Check sheet for the modelled part. Datum: model origin and axes. Units: mm. A direction names the side the tool comes from. Round coordinates to 2 decimals unless told otherwise and drop trailing zeros. Order: outer loops, then holes, each group sorted by start corner. A loop starts at its lowest first (then second) coordinate and runs counter-clockwise, first axis right, second up.
Q1. Cross-section at A-A on z = -26. Record the cut outline in (x, y), then the cut area to 3 significant figures.
Q2. Mould release check, pull along X, two halves, no side actions. Record for faces 4 (the flat face through (21, 2, 32)), 5 (the flat face through (26, 1, 1)), 6 (the flat face through (-17, 1, 1)), 7 (the flat face through (-2, 3, -1)): +X half, -X half, draft (parallel to the pull), parting line (faces both ways), or undercut.
Q3. Cross-section at D-D on z = 3.5. Record the cut outline in (x, y).
Q4. Scan lines: probe 1 along X at (y, z) = (1.3, -31); probe 2 along X at (y, z) = (2.6, 32); probe 3 along X at (y, z) = (0.75, 15). Record each from-to range of solid material in increasing order.
Q5. Depth check by flat-ended pin: P1, Ø1.1, axis at x = -26, y = 2.5, coming from the -Z side; P2, Ø2.5, axis at x = 23, z = 33, coming from the -Y side; P3, Ø0.8, axis at y = 2.5, z = -31.5, coming from the -X side. Enter the tip coordinate at first touch or a pass-through.
Q6. Cross-section at C-C on y = 0.95. Record the cut outline in (x, z).
Q7. Set-up check for faces 1 (the cylindrical face through (3.138, 1.479, 11.853)), 2 (the flat face through (-23, 2, -1)), 3 (the cylindrical face through (24.27, 0.99, 30.23)): record each of +Z, -Z, +X, -X, +Y, -Y from which the full face is reachable in a straight line by a thin tool's end or side.
Q8. Cross-section at B-B on x = 15. Record the cut outline in (y, z).
from build123d import *

# Parameters (mm, degrees)
ESQUISSE1_R             = 1.7
ESQUISSE1_R_2           = 3.15
ESQUISSE1_R_3           = 1.4
BOSS_EXTRU_3_DEPTH      = 3
ESQUISSE1_5_R           = 1.4
ESQUISSE1_5_R_2         = 2.4
ENL_V_MAT_EXTRU_7_DEPTH = 2


with BuildPart() as part:
    # Esquisse1 → Boss.-Extru.3 (new body)
    with BuildSketch(Plane(origin=(0, 0, 0), x_dir=(1, 0, 0), z_dir=(0, 1, 0))):
        Polygon((-21, 36), (-21, 28), (-29, 28), (-29, -36), (26, -36), (26, 36), align=None)
        with Locations(Location((15, 31, 0), (0, 0, 270))):
            Circle(ESQUISSE1_R, mode=Mode.SUBTRACT)
        with Locations(Location((3, -15, 0), (0, 0, 270))):
            Circle(ESQUISSE1_R_2, mode=Mode.SUBTRACT)
        with Locations(Location((-15, 31, 0), (0, 0, 270))):
            Circle(ESQUISSE1_R, mode=Mode.SUBTRACT)
        with Locations(Location((-26.347888471, 26, 0), (0, 0, 270))):
            Circle(ESQUISSE1_R_3, mode=Mode.SUBTRACT)
        with Locations(Location((22.652111529, 26, 0), (0, 0, 270))):
            Circle(ESQUISSE1_R_3, mode=Mode.SUBTRACT)
        with Locations(Location((22.652111529, -32, 0), (0, 0, 270))):
            Circle(ESQUISSE1_R_3, mode=Mode.SUBTRACT)
        with Locations(Location((-26.347888471, -32, 0), (0, 0, 270))):
            Circle(ESQUISSE1_R_3, mode=Mode.SUBTRACT)
    extrude(amount=BOSS_EXTRU_3_DEPTH)

    # Esquisse1_5 → Enl_v. mat.-Extru.7 (cut)
    # profile 1 of 3: a face of its own
    with BuildSketch(Plane(origin=(0, 0, 0), x_dir=(1, 0, 0), z_dir=(0, 1, 0))):
        Polygon((-17, 36), (-21, 36), (-21, 28), (-29, 28), (-29, -36), (-17, -36), align=None)
        with Locations(Location((-26.347888471, 26, 0), (0, 0, 270))):
            Circle(ESQUISSE1_5_R, mode=Mode.SUBTRACT)
        with Locations(Location((-26.347888471, -32, 0), (0, 0, 270))):
            Circle(ESQUISSE1_5_R, mode=Mode.SUBTRACT)
    # profile 2 of 3: a face of its own
    with BuildSketch(Plane(origin=(0, 0, 0), x_dir=(1, 0, 0), z_dir=(0, 1, 0))):
        with Locations(Location((22.652111529, 26, 0), (0, 0, 270))):
            Circle(ESQUISSE1_5_R_2)
        with Locations(Location((22.652111529, 26, 0), (0, 0, 270))):
            Circle(ESQUISSE1_5_R, mode=Mode.SUBTRACT)
    # profile 3 of 3: a face of its own
    with BuildSketch(Plane(origin=(0, 0, 0), x_dir=(1, 0, 0), z_dir=(0, 1, 0))):
        with Locations(Location((22.652111529, -32, 0), (0, 0, 270))):
            Circle(ESQUISSE1_5_R_2)
        with Locations(Location((22.652111529, -32, 0), (0, 0, 270))):
            Circle(ESQUISSE1_5_R, mode=Mode.SUBTRACT)
    extrude(amount=ENL_V_MAT_EXTRU_7_DEPTH, mode=Mode.SUBTRACT)


solid = part.part
Results found:
1. outline: (-29, 2) - (-27.75, 2) - (-27.75, 3) - (-29, 3) - close; (-24.95, 2) - (-17, 2) - (-17, 0) - (20.25, 0) - (20.25, 2) - (21.25, 2) - (21.25, 3) - (-24.95, 3) - close; (24.05, 2) - (25.05, 2) - (25.05, 0) - (26, 0) - (26, 3) - (24.05, 3) - close
1. area: 126 mm2
2. face 4: undercut
2. face 5: +X half
2. face 6: -X half
2. face 7: draft
3. outline: (-29, 2) - (-17, 2) - (-17, 0) - (26, 0) - (26, 3) - (-29, 3) - close
4. probe 1: x = -17 to -16.7, -13.3 to 13.3, 16.7 to 26
4. probe 2: x = -29 to -27.75, -24.95 to 21.25, 24.05 to 26
4. probe 3: x = -17 to -0.15, 6.15 to 26
5. P1: stops at z = -28
5. P2: stops at y = 2
5. P3: stops at x = -21
6. outline: (-17, -36) - (26, -36) - (26, 36) - (-17, 36) - close; hole circle Ø3.4 at (-15, -31); hole circle Ø6.3 at (3, 15); hole circle Ø3.4 at (15, -31); hole circle Ø4.8 at (22.65, -26); hole circle Ø4.8 at (22.65, 32)
7. face 1: +Y, -Y
7. face 2: +Z, -Z, -X, -Y
7. face 3: -Y
8. outline: (0, -36) - (3, -36) - (3, -32.7) - (0, -32.7) - close; (0, -29.3) - (3, -29.3) - (3, 36) - (0, 36) - close
